Model file for the job. Use its own axes, mm. A direction names the side the tool comes from. Coordinates: 2 decimals unless noted, no trailing zeros. Write each loop counter-clockwise with the first axis right and the second up, starting at its lowest first coordinate (ties: lowest second). Pieces come first, ordered by that corner, then holes. Notation, with made-up numbers: M 55,27.25 L 75,27.25 A23 cw 75,49.25 Z; hole C 80,61.5 d3. An arc over 180 degrees is marked long. Use CSV: the item, a comma, the result in double quotes. Start each with the question number.
from build123d import *

# Parameters (mm, degrees)
SKETCH1_W           = 140
SKETCH1_H           = 3
BOSS_EXTRUDE1_DEPTH = 95
CUT_EXTRUDE1_DEPTH  = 95
SKETCH4_W           = 45
SKETCH4_H           = 50
CUT_EXTRUDE3_DEPTH  = 10


with BuildPart() as part:
    # Sketch1 → Boss-Extrude1 (new body)
    with BuildSketch(Plane(origin=(0, 0, 0), x_dir=(1, 0, 0), z_dir=(0, 1, 0))):
        Rectangle(SKETCH1_W, SKETCH1_H)
    extrude(amount=BOSS_EXTRUDE1_DEPTH)

    # Sketch 377 → Cut-Extrude1 (cut)
    with BuildSketch(Plane(origin=(0, 95, 0), x_dir=(1, 0, 0), z_dir=(0, 1, 0))):
        Polygon((70, -1.5), (70, 1.5), (67, 1.5), align=None)
        Polygon((-70, -1.5), (-70, 1.5), (-67, 1.5), align=None)
    extrude(amount=-CUT_EXTRUDE1_DEPTH, mode=Mode.SUBTRACT)

    # Sketch4 → Cut-Extrude3 (cut)
    with BuildSketch(Plane.XY.offset(1.5)):
        with Locations((42.5, 25)):
            Rectangle(SKETCH4_W, SKETCH4_H)
    extrude(amount=-CUT_EXTRUDE3_DEPTH, mode=Mode.SUBTRACT)


solid = part.part
1) Wall check: L1, parallel to X at y = 32, z = 1.45; L2, parallel to X at y = 47.5, z = 0.3; L3, parallel to Y at x = 53.5, z = 0.45. Give the ranges that are in metal, low to high. Write a range as [from, to].
2) Two-plate mould, pull along X, no slides. Class faces 1 (the face through (68.5, 48.2, 0)), 2 (the face through (-1, 95, 0)), 3 (the face through (65, 25, 0)): pulls with the +X half, pulls with the -X half, needs draft (parallel to the pull), parting line crosses it, or undercut.
3) Drop a flat-ended pin along its axis: P1, Ø1.5, axis at y = 22.5, z = -0.5, coming from the +X side. Give the stop position or say it passes through.
4) Band-saw the part on B-B on z = -0.45. List the corners of the cut face in (x, y).
5) Band-saw the part on A-A on y = 46. List the corners of the cut face in (x, z), then the cut area to 3 significant figures.
6) Band-saw the part on C-C on x = 51.5. List the corners of the cut face in (y, z), then the cut area to 3 significant figures.
7) Band-saw the part on D-D on y = 71. List the corners of the cut face in (x, z), then the cut area to 3 significant figures.
8) Tool access for faces 4 (the face through (20, 25, 0)), 5 (the face through (-68.5, 48.2, 0)): list every direction of +Z, -Z, +X, -X, +Y, -Y with a clear straight run to the whole face (end or side of a thin tool).
Findings below:
1,L1,"x = [-69.95, 20], [65, 69.95]"
1,L2,"x = [-68.8, 20], [65, 68.8]"
1,L3,"y = [50, 95]"
2,face 1,"pulls with the +X half"
2,face 2,"needs draft"
2,face 3,"undercut"
3,P1,"stops at x = 68.75"
4,outline,"M -68.05,0 L 20,0 L 20,50 L 65,50 L 65,0 L 68.05,0 L 68.05,95 L -68.05,95 Z"
5,outline,"M -70,1.5 L -67,-1.5 L 20,-1.5 L 20,1.5 Z; M 65,-1.5 L 67,-1.5 L 70,1.5 L 65,1.5 Z"
5,area,"276 mm2"
6,outline,"M 50,-1.5 L 95,-1.5 L 95,1.5 L 50,1.5 Z"
6,area,"135 mm2"
7,outline,"M -70,1.5 L -67,-1.5 L 67,-1.5 L 70,1.5 Z"
7,area,"411 mm2"
8,face 4,"+Z, -Z, -Y"
8,face 5,"-Z, -X, +Y, -Y"
